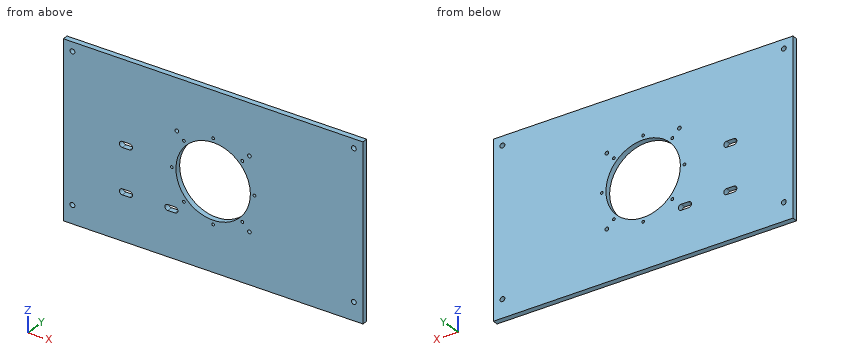
from build123d import *

# Parameters (mm, degrees)
SKETCH1_W                = 330
SKETCH1_H                = 192
BOSS_EXTRUDE1_DEPTH      = 6
CUT_EXTRUDE1_DEPTH       = 382.837661841
CUT_EXTRUDE1_DEPTH_BACK  = 382.837661841
SKETCH2_R                = 1.5
SKETCH3_R                = 41
CUT_EXTRUDE2_DEPTH       = 382.837661841
CUT_EXTRUDE5_DEPTH       = 10
SKETCH11_R               = 2
CUT_EXTRUDE6_DEPTH       = 10
M5_CLEARANCE_HOLE1_D     = 5.3
M5_CLEARANCE_HOLE1_DEPTH = 11.94
M5_CLEARANCE_HOLE1_TIP   = 1.59228064


with BuildPart() as part:
    # Sketch1 → Boss-Extrude1 (new body)
    with BuildSketch(Plane(origin=(0, 0, 0), x_dir=(1, 0, 0), z_dir=(0, 1, 0))):
        with Locations((165, 96)):
            Rectangle(SKETCH1_W, SKETCH1_H)
    extrude(amount=BOSS_EXTRUDE1_DEPTH)

    # Sketch2 → Cut-Extrude1 (cut, two sides: drawn at the far end of the back side and taken through both)
    with BuildSketch(Plane(origin=(0, 6, 0), x_dir=(1, 0, 0), z_dir=(0, 1, 0)).offset(-CUT_EXTRUDE1_DEPTH_BACK)):
        with Locations(Location((165, 141.5, 0), (0, 0, 270))):
            Circle(SKETCH2_R)
        with Locations(Location((197.173358544, 128.173358544, 0), (0, 0, 270))):
            Circle(SKETCH2_R)
        with Locations(Location((210.5, 96, 0), (0, 0, 270))):
            Circle(SKETCH2_R)
        with Locations(Location((165, 50.5, 0), (0, 0, 270))):
            Circle(SKETCH2_R)
        with Locations(Location((132.826641456, 63.826641456, 0), (0, 0, 270))):
            Circle(SKETCH2_R)
        with Locations(Location((119.5, 96, 0), (0, 0, 270))):
            Circle(SKETCH2_R)
        with Locations(Location((132.826641456, 128.173358544, 0), (0, 0, 270))):
            Circle(SKETCH2_R)
        with Locations(Location((197.173358544, 63.826641456, 0), (0, 0, 270))):
            Circle(SKETCH2_R)
    extrude(amount=CUT_EXTRUDE1_DEPTH + CUT_EXTRUDE1_DEPTH_BACK, mode=Mode.SUBTRACT)

    # Sketch3 → Cut-Extrude2 (cut, through all)
    with BuildSketch(Plane(origin=(0, 6, 0), x_dir=(1, 0, 0), z_dir=(0, 1, 0))):
        with Locations(Location((165, 96, 0), (0, 0, 270))):
            Circle(SKETCH3_R)
    extrude(amount=-CUT_EXTRUDE2_DEPTH, mode=Mode.SUBTRACT)

    # Sketch10 → Cut-Extrude5 (cut)
    with BuildSketch(Plane.XZ):
        with BuildLine():
            Line((123, -136.8), (115, -136.8))
            ThreePointArc((115, -136.8), (111.8, -140), (115, -143.2))
            Line((115, -143.2), (123, -143.2))
            ThreePointArc((123, -143.2), (126.2, -140), (123, -136.8))
        make_face()
        with BuildLine():
            Line((73, -136.8), (65, -136.8))
            ThreePointArc((65, -136.8), (61.8, -140), (65, -143.2))
            Line((65, -143.2), (73, -143.2))
            ThreePointArc((73, -143.2), (76.2, -140), (73, -136.8))
        make_face()
        with BuildLine():
            Line((73, -86.8), (65, -86.8))
            ThreePointArc((65, -86.8), (61.8, -90), (65, -93.2))
            Line((65, -93.2), (73, -93.2))
            ThreePointArc((73, -93.2), (76.2, -90), (73, -86.8))
        make_face()
    extrude(amount=-CUT_EXTRUDE5_DEPTH, mode=Mode.SUBTRACT)

    # Sketch11 → Cut-Extrude6 (cut)
    with BuildSketch(Plane.XZ):
        with Locations(Location((125, -56, 0), (0, 0, 270))):
            Circle(SKETCH11_R)
        with Locations(Location((205, -56, 0), (0, 0, 270))):
            Circle(SKETCH11_R)
        with Locations(Location((205, -136, 0), (0, 0, 270))):
            Circle(SKETCH11_R)
    extrude(amount=-CUT_EXTRUDE6_DEPTH, mode=Mode.SUBTRACT)

    # M5 Clearance Hole1
    with Locations(Plane(origin=(0, 6, 0), x_dir=(1, 0, 0), z_dir=(0, 1, 0))):
        with Locations((10, 172), (10, 10), (320, 10), (320, 172)):
            Hole(M5_CLEARANCE_HOLE1_D / 2, depth=M5_CLEARANCE_HOLE1_DEPTH)
            with Locations((0, 0, -(M5_CLEARANCE_HOLE1_DEPTH + M5_CLEARANCE_HOLE1_TIP / 2))):  # 118° drill point
                Cone(0, M5_CLEARANCE_HOLE1_D / 2, M5_CLEARANCE_HOLE1_TIP, mode=Mode.SUBTRACT)


solid = part.part
Here's how the part is built. I have some questions about the finished solid (model axes, mm). Coordinates: 2 decimals unless noted, no trailing zeros. Write each loop counter-clockwise with the first axis right and the second up, starting at its lowest first coordinate (ties: lowest second). Pieces come first, ordered by that corner, then holes. Notation, with made-up numbers: (-22.75, 47.25) - (27.25, 47.25) arc R16 cw to (27.25, 70.25) - close; hole circle Ø3 at (16.5, -29). An arc over 180 degrees is marked (long way). Use one line per item in the form item = value.
1) I need wall thicknesses on line 1 (X direction, y = 3.1, z = -10); line 2 (Z direction, x = 320, y = 2.4); line 3 (X direction, y = 3.45, z = -96). Which ranges of each line are inside material? Lowest first, please.
Solved:
line_1 = 0 to 7.35, 12.65 to 317.35, 322.65 to 330
line_2 = -192 to -174.65, -169.35 to -12.65, -7.35 to 0
line_3 = 0 to 118, 121 to 124, 206 to 209, 212 to 330
2) I'm going to push a flat-ended pin straight in: P1, Ø3, axis at x = 205, z = -56, coming from the -Y side. Where does the tip first touch, or does it pass through?
Solved:
P1 = through
3) Suppose I cut it at A-A, the plane z = -90. Write out the boundary of the cut face in (x, y), plus the area to 3 significant figures.
Solved:
outline = (0, 0) - (61.8, 0) - (61.8, 6) - (0, 6) - close; (76.2, 0) - (124.44, 0) - (124.44, 6) - (76.2, 6) - close; (205.56, 0) - (330, 0) - (330, 6) - (205.56, 6) - close
area = 1,410 mm2
4) Suppose I cut it at C-C, the plane y = 2. Give the number of separate pieces and of enclosed holes in the cut face, plus the area to 3 significant figures.
Solved:
separate_pieces = 1
enclosed_holes = 19
area = 57,600 mm2
5) Suppose I cut it at B-B, the plane x = 186. Write out the boundary of the cut face in (y, z).
Solved:
outline = (0, -192) - (6, -192) - (6, -131.21) - (0, -131.21) - close; (0, -60.79) - (6, -60.79) - (6, 0) - (0, 0) - close
